Autodesk Inventor part; units mm, degrees
ref_plane "YZ Plane" through (0, 0, 0) normal (1, 0, 0) x (0, 1, 0)
ref_plane "XZ Plane" through (0, 0, 0) normal (0, 1, 0) x (-1, 0, 0)
ref_plane "XY Plane" through (0, 0, 0) normal (0, 0, 1) x (1, 0, 0)
sketch "Sketch1" plane through (0, 0, 0) normal (0, 0, 1) x (1, 0, 0)
  arc A0 (-31.1131, 4.9219) -> (31.1131, 4.9219) centre (0, 0) ccw
  line L0 (-31.1131, 4.9219) -> (-36.1667, 4.9219)
  line L1 (31.1131, 4.9219) -> (36.1836, 4.9349)
  line L2 (31.1131, 4.9219) -> (36.1836, 4.9349) construction
  line L3 (5.0676, -36.5047) -> (5.0676, -51.5047)
  line L4 (5.0676, -51.5047) -> (-4.9324, -51.5047)
  line L5 (-4.9324, -51.5047) -> (-4.9324, -36.5047)
  line L6 (-4.9324, -36.5047) -> (-4.9324, -36.1653)
  line L7 (5.0676, -36.5047) -> (5.0676, -36.1653)
  arc A1 (-36.1667, 4.9219) -> (-4.9324, -36.1653) centre (0, 0) ccw
  arc A2 (5.0676, -36.1653) -> (36.1836, 4.9349) centre (0, 0) ccw
  dimension "d0" = 63
  dimension "d5" = 10
  dimension "d6" = 15
extrude "Extrusion1" add sketch "Sketch1" along normal blind 5
properties part number "Clip_TestFitV1"
Can you work these out from the model? Positions are in its coordinate system, mm. A direction names the side the tool comes from. Round coordinates to 2 decimals unless told otherwise and drop trailing zeros. Loops run counter-clockwise (first coordinate to the right, second up) from the corner with the lowest first, then second, coordinate; pieces in that order, holes last. Notation, with made-up numbers: M 15,50.25 L 44,50.25 A18 cw 44,63.25 Z; hole C -12.75,-2 d11. An arc over 180 degrees is marked long. Answer as a JSON object with one key per item and string values. Group by question number.
Q1. Imagine slicing it at C-C, the plane x = 0. Please give me the cut outline in (y, z).
Q2. Please list where these lines run through material, in increasing order: L1, parallel to X at y = 0, z = 2.6; L2, parallel to X at y = -22.5, z = 1.75; L3, parallel to Y at x = -6.5, z = 1.1.
Q3. Will these pins go through, and if not, where does the flat tip stop? pin 1 (3 mm diameter, centred on x = -19.5, z = 3.5, fed in from -Y); pin 2 (1.5 mm diameter, centred on x = -12.5, z = 3.5, fed in from +Y); pin 3 (1.5 mm diameter, centred on y = -37, z = 2, fed in from -X).
Q4. Imagine slicing it at D-D, the plane x = -7.5. Please give me the cut outline in (y, z).
Q5. Imagine slicing it at B-B, the plane y = -10. Please give me the cut outline in (x, z).
Q6. Imagine slicing it at A-A, the plane y = 0. Please give me the cut outline in (x, z), then the cut area to 3 significant figures.
Q7. We'd pull the mould along Y, two halves only. Please class faces 4 (the cylindrical face through (0.76, -31.49, 2.46)), 5 (the flat face through (0, -51.505, 2)), 6 (the flat face through (-34, 4.922, 2)): +Y half, -Y half, draft (parallel to the pull), parting line (faces both ways), or undercut.
Q8. On a 3-axis mill with a long thin cutter (end or side, diameter ignored), from which of +Z, -Z, +X, -X, +Y, -Y can I reach the whole of each face in a straight line? I mean faces 1 (the flat face through (0, -32, 5)), 2 (the flat face through (-4.932, -44, 2)), 3 (the flat face through (5.068, -44, 2)). Say none if no direction works.
Findings:
{
 "1": {"outline": "M -51.5,0 L -31.5,0 L -31.5,5 L -51.5,5 Z"},
 "2": {"L1": "x = -36.5 to -31.5, 31.5 to 36.52", "L2": "x = -28.74 to -22.05, 22.05 to 28.76", "L3": "y = -35.92 to -30.82"},
 "3": {"pin 1": "stops at y = -31.75", "pin 2": "stops at y = -28.58", "pin 3": "stops at x = -4.93"},
 "4": {"outline": "M -35.72,0 L -30.59,0 L -30.59,5 L -35.72,5 Z"},
 "5": {"outline": "M -35.1,0 L -29.87,0 L -29.87,5 L -35.1,5 Z; M 29.87,0 L 35.12,0 L 35.12,5 L 29.87,5 Z"},
 "6": {"outline": "M -36.5,0 L -31.5,0 L -31.5,5 L -36.5,5 Z; M 31.5,0 L 36.52,0 L 36.52,5 L 31.5,5 Z", "area": "50.1 mm2"},
 "7": {"face 4": "undercut", "face 5": "-Y half", "face 6": "+Y half"},
 "8": {"face 1": "+Z, +X, -X, +Y, -Y", "face 2": "+Z, -Z, -X, -Y", "face 3": "+Z, -Z, +X, -Y"}
}
